Verification items for the finished model (mm, model axes). Face numbers are marked on the shaded views. A direction names the side the tool comes from. Round coordinates to 2 decimals unless told otherwise and drop trailing zeros. Order: outer loops, then holes, each group sorted by start corner. A loop starts at its lowest first (then second) coordinate and runs counter-clockwise, first axis right, second up. Notation, with made-up numbers: (-33.75, -23) -> (-6.75, -23) arc R12 ccw to (-6.75, -4) -> close; hole circle Ø10 at (-18, 33). An arc over 180 degrees is marked (long way). Put each result on its own line as item: value.
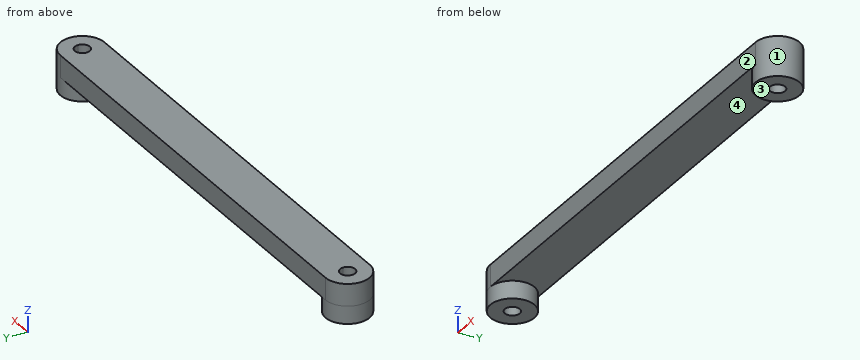
```python
from build123d import *

# Parameters (mm, degrees)
F0_R     = 1.7
F1_DEPTH = 5
F2_R     = 5
F2_R_2   = 1.7
F3_DEPTH = 4


with BuildPart() as f1:
    # F0 (on Top) → F1 (new body)
    with BuildSketch(Plane.XY):
        with BuildLine():
            Line((-50.605015, -5), (50.605015, -5))
            ThreePointArc((50.605015, -5), (55.605015, 0), (50.605015, 5))
            Line((50.605015, 5), (-50.605015, 5))
            ThreePointArc((-50.605015, 5), (-55.605015, 0), (-50.605015, -5))
        make_face()
        with Locations((-50.605015, 0)):
            Circle(F0_R, mode=Mode.SUBTRACT)
        with Locations((50.605015, 0)):
            Circle(F0_R, mode=Mode.SUBTRACT)
    extrude(amount=F1_DEPTH)

    # F2 (on face) → F3 (join)
    with BuildSketch(Plane(origin=(0, 0, 0), x_dir=(1, 0, 0), z_dir=(0, 0, -1))):
        with Locations((-50.605015, 0)):
            Circle(F2_R)
        with Locations((-50.605015, 0)):
            Circle(F2_R_2, mode=Mode.SUBTRACT)
    extrude(amount=F3_DEPTH)

    # F4: F1 across plane


with BuildPart() as f1_1:
    add(f1.part)
    add(f1.part.mirror(Plane.YZ))


solid = f1_1.part
```
Item 1: Depth check by flat-ended pin: pin 1 Ø4 at (y, z) = (4, -2.5) entering from -X; pin 2 Ø1 at (y, z) = (3.5, 0.5) entering from -X (3 decimals); pin 3 Ø3 at (x, y) = (-24, -2) entering from -Z. Enter the tip coordinate at first touch or a pass-through.
Geometry check:
pin 1: x = -55.19
pin 2: x = -54.605
pin 3: z = 0
Item 2: Sectioned sample at A-A, the plane z = -3. Record the boundary of the cut face in (x, y).
Geometry check:
outline: circle Ø10 at (-50.61, 0); circle Ø10 at (50.61, 0); hole circle Ø3.4 at (-50.61, 0); hole circle Ø3.4 at (50.61, 0)
Item 3: Release check for a two-part mould opening along X. For the marked faces 3 and 4 record: pulls with the +X half, pulls with the -X half, needs draft (parallel to the pull), parting line crosses it, or undercut.
Geometry check:
face 3: needs draft
face 4: undercut
Item 4: Material ranges on line 1 along X through (y, z) = (0, -0.75); line 2 along X through (y, z) = (0.5, -2.25); line 3 along X through (y, z) = (-1.5, 1.75), recorded low to high.
Geometry check:
line 1: -55.61 to -52.31, -48.91 to -45.61, 45.61 to 48.91, 52.31 to 55.61
line 2: -55.58 to -52.23, -48.98 to -45.63, 45.63 to 48.98, 52.23 to 55.58
line 3: -55.37 to -51.41, -49.81 to 49.81, 51.41 to 55.37
Item 5: Sectioned sample at C-C, the plane x = -10. Record the boundary of the cut face in (y, z).
Geometry check:
outline: (-5, 0) -> (5, 0) -> (5, 5) -> (-5, 5) -> close
Item 6: Sectioned sample at B-B, the plane z = 2. Record the boundary of the cut face in (x, y).
Geometry check:
outline: (-50.61, -5) -> (50.61, -5) arc R5 ccw to (50.61, 5) -> (-50.61, 5) arc R5 ccw to start; hole circle Ø3.4 at (-50.61, 0); hole circle Ø3.4 at (50.61, 0)
Item 7: Tool access check on the marked faces 1 and 2. Record the directions out of +Z, -Z, +X, -X, +Y, -Y that give a thin tool (end or side, any length) a straight path to the whole face; none if there is none.
Geometry check:
face 1: -Z
face 2: +Z, -Z, +X, -X, -Y
